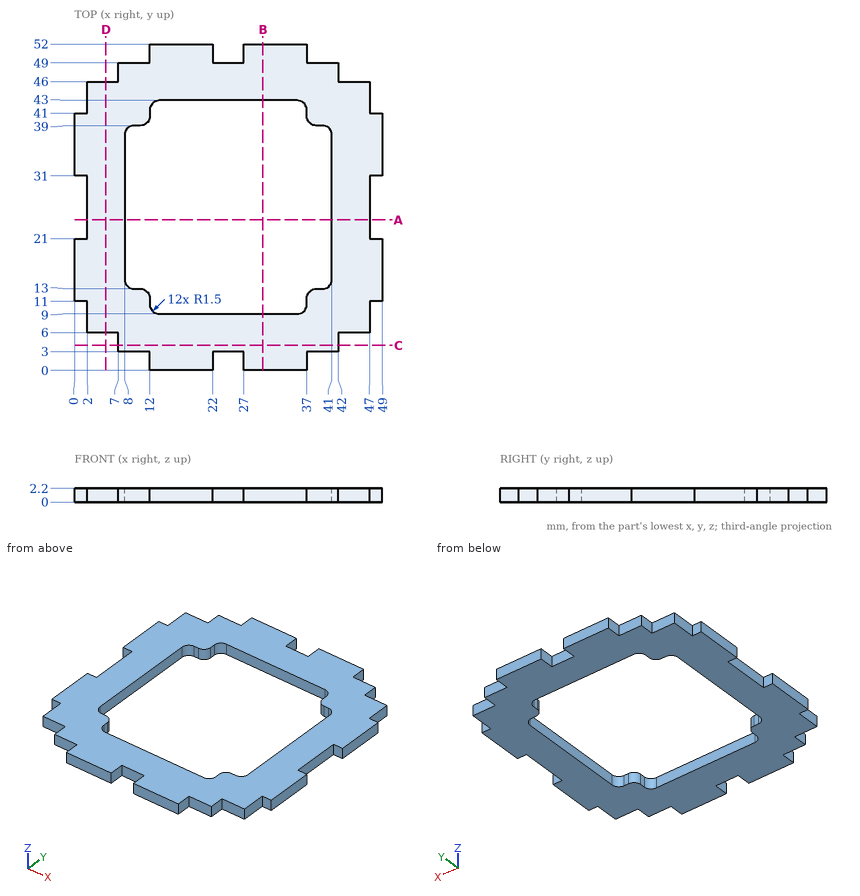
Could you check a few things on this drawing? It's one solid part, dimensions in mm from its lowest x, y, z. Coordinates: 2 decimals unless noted, no trailing zeros. Order: outer loops, then holes, each group sorted by start corner. A loop starts at its lowest first (then second) coordinate and runs counter-clockwise, first axis right, second up. Notation, with made-up numbers: M 67,-26.5 L 102,-26.5 A26 cw 102,7.5 Z; hole C 19,19.5 d10. An arc over 180 degrees is marked long. Use one line per item in the form item = value. Start each with the question number.
1. For pin 1 (0.7 mm diameter, centred on x = 39.5, z = 1.5, fed in from -Y); pin 2 (0.7 mm diameter, centred on y = 1, z = 1, fed in from +X); pin 3 (0.7 mm diameter, centred on x = 43.5, z = 1.5, fed in from -Y), each with a flat end and sliding along its axis, tell me the tip position at first contact or that it passes through.
2. Suppose I cut it at C-C on y = 4. Write out the boundary of the cut face in (x, z), then the cut area to 3 significant figures.
3. Suppose I cut it at D-D on x = 5. Write out the boundary of the cut face in (y, z), then the cut area to 3 significant figures.
4. Please list where these lines run through material, in increasing order: line 1 (X direction, y = 26.5, z = 0.95); line 2 (Y direction, x = 21.5, z = 1.3); line 3 (X direction, y = 20, z = 0.55).
5. Suppose I cut it at B-B on x = 30. Write out the boundary of the cut face in (y, z).
6. Suppose I cut it at A-A on y = 24. Write out the boundary of the cut face in (x, z).
Geometry says:
q1.pin_1 = 3
q1.pin_2 = 37
q1.pin_3 = 6
q2.outline = M 7,0 L 42,0 L 42,2.2 L 7,2.2 Z
q2.area = 77.0 mm^2
q3.outline = M 6,0 L 46,0 L 46,2.2 L 6,2.2 Z
q3.area = 88.0 mm^2
q4.line_1 = 2 to 8, 41 to 47
q4.line_2 = 0 to 9, 43 to 52
q4.line_3 = 0 to 8, 41 to 49
q5.outline = M 0,0 L 9,0 L 9,2.2 L 0,2.2 Z; M 43,0 L 52,0 L 52,2.2 L 43,2.2 Z
q6.outline = M 2,0 L 8,0 L 8,2.2 L 2,2.2 Z; M 41,0 L 47,0 L 47,2.2 L 41,2.2 Z
